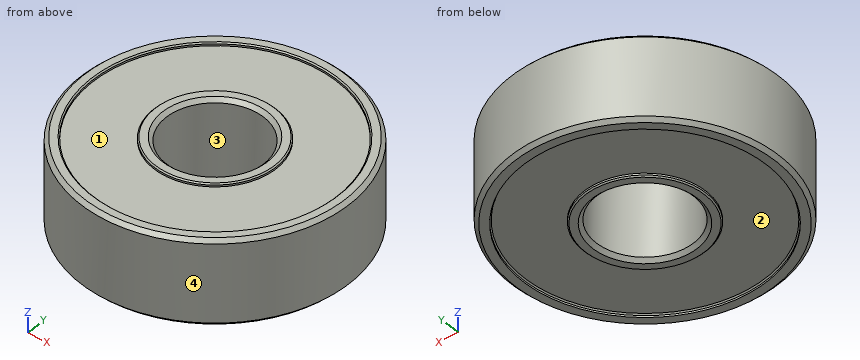
```python
from build123d import *

# Parameters (mm, degrees)
SKETCH1_R             = 11
SKETCH1_R_2           = 10
BOSS_EXTRUDE1_DEPTH   = 3.5
SKETCH1_R_3           = 5
SKETCH1_R_4           = 4
BOSS_EXTRUDE1_2_DEPTH = 3.5
SKETCH1_3_R           = 10
SKETCH1_3_R_2         = 5
BOSS_EXTRUDE2_DEPTH   = 3.25
CHAMFER1_SIZE         = 0.3
CHAMFER2_SIZE         = 0.1


with BuildPart() as part:
    # Sketch1 → Boss-Extrude1 (new body, symmetric)
    with BuildSketch(Plane.XY):
        Circle(SKETCH1_R)
        Circle(SKETCH1_R_2, mode=Mode.SUBTRACT)
    extrude(amount=BOSS_EXTRUDE1_DEPTH, both=True)



with BuildPart() as body_2:
    # Sketch1 → Boss-Extrude1 2 (new body, symmetric)
    with BuildSketch(Plane.XY):
        Circle(SKETCH1_R_3)
        Circle(SKETCH1_R_4, mode=Mode.SUBTRACT)
    extrude(amount=BOSS_EXTRUDE1_2_DEPTH, both=True)


with BuildPart() as part_1:
    add(part.part)

    add(body_2.part)  # Boss-Extrude2 merges body 2
    # Sketch1_3 → Boss-Extrude2 (add, symmetric)
    with BuildSketch(Plane.XY):
        Circle(SKETCH1_3_R)
        Circle(SKETCH1_3_R_2, mode=Mode.SUBTRACT)
    extrude(amount=BOSS_EXTRUDE2_DEPTH, both=True)

    # Chamfer1
    chamfer1_edges = [part_1.edges().sort_by_distance(p)[0] for p in [
        (-11, 0, 3.5),
        (-4, 0, 3.5),
        (-4, 0, -3.5),
        (-11, 0, -3.5),
    ]]
    chamfer(chamfer1_edges, length=CHAMFER1_SIZE)

    # Chamfer2
    chamfer2_edges = [part_1.edges().sort_by_distance(p)[0] for p in [
        (-10, 0, -3.25),
        (-5, 0, -3.5),
        (-5, 0, 3.5),
        (-10, 0, 3.5),
    ]]
    chamfer(chamfer2_edges, length=CHAMFER2_SIZE)


solid = part_1.part
```
Read the model definition and answer for the solid it produces. Units are mm, in the model's axes. Face numbers are marked on the shaded views. A direction names the side the tool comes from. Coordinates: 2 decimals unless noted, no trailing zeros. Loops run counter-clockwise (first coordinate to the right, second up) from the corner with the lowest first, then second, coordinate; pieces in that order, holes last.
(1) The part is cut by section A-A (z = -2). Determine the outline of the cut face in (x, y), and give its area (3 significant figures).
Solution:
outline: circle Ø22 at (0, 0); hole circle Ø8 at (0, 0)
area: 330 mm2
(2) The mould has two halves that part along X. Classify the marked faces 3 and 4: released by +X, released by -X, zero draft, split by the parting line, or undercut.
Solution:
face 3: undercut
face 4: split by the parting line
(3) A flat-ended cylindrical pin translates along its axis: pin 1 Ø1 at (x, y) = (3, -5.5) entering from +Z. Find the tip coordinate at first contact, or state that the pin passes through.
Solution:
pin 1: stops at z = 3.25
(4) Consider line 1 along Y through (x, z) = (0, 1.5); line 2 along Y through (x, z) = (-1.5, -2); line 3 along Z through (x, y) = (-0.75, 7). Determine where each line is inside the solid, lowest interval first.
Solution:
line 1: y = -11 to -4, 4 to 11
line 2: y = -10.9 to -3.71, 3.71 to 10.9
line 3: z = -3.25 to 3.25
(5) A tool of negligible diameter and unlimited length cuts with its end or side. For the marked faces 1 and 2, from which of +Z, -Z, +X, -X, +Y, -Y can it reach the whole face along a straight path? Write none if from no direction.
Solution:
face 1: +Z
face 2: -Z
